Verification items for the finished model (mm, model axes). Round coordinates to 2 decimals unless told otherwise and drop trailing zeros. Order: outer loops, then holes, each group sorted by start corner. A loop starts at its lowest first (then second) coordinate and runs counter-clockwise, first axis right, second up. Notation, with made-up numbers: (10, 56.5) -> (18, 56.5) arc R30 cw to (18, 91.5) -> close; hole circle Ø11 at (58.25, 46.5). An arc over 180 degrees is marked (long way). Answer in a Markdown table with one row per item. Add a question column.
```python
from build123d import *

# Parameters (mm, degrees)
BOSS_EXTRUDE1_DEPTH = 3.175
CUT_EXTRUDE1_REACH  = 275.585
SKETCH2_W           = 1.6256
SKETCH2_H           = 4.7244


with BuildPart() as part:
    # Sketch1 → Boss-Extrude1 (new body)
    with BuildSketch(Plane(origin=(0, 0, 0), x_dir=(1, 0, 0), z_dir=(0, 1, 0))):
        Polygon((171.45, 101.6), (254, 101.6), (254, 0), (0, 0), (0, 101.6), (82.55, 101.6), (82.55, 76.2), (171.45, 76.2), align=None)
    extrude(amount=BOSS_EXTRUDE1_DEPTH)

    # Sketch2 → Cut-Extrude1 (cut, up to next)
    with BuildSketch(Plane(origin=(0, 3.175, 0), x_dir=(-1, 0, 0), z_dir=(0, 1, 0)), mode=Mode.PRIVATE) as cut_extrude1_sk1:
        with Locations((-97.742468943, -73.8378)):
            Rectangle(SKETCH2_W, SKETCH2_H)
    cut_extrude1_tool1 = extrude(cut_extrude1_sk1.sketch, amount=-CUT_EXTRUDE1_REACH, mode=Mode.PRIVATE) & part.part
    # Sketch2 → Cut-Extrude1 (cut, up to next)
    with BuildSketch(Plane(origin=(0, 3.175, 0), x_dir=(-1, 0, 0), z_dir=(0, 1, 0)), mode=Mode.PRIVATE) as cut_extrude1_sk2:
        Polygon((-113.996008389, -76.2), (-115.621608389, -76.2), (-115.621608389, -71.4756), (-113.996008389, -71.4756), (-113.996008389, -59.055), (-112.370408389, -59.055), (-112.370408389, -76.2), align=None)
    cut_extrude1_tool2 = extrude(cut_extrude1_sk2.sketch, amount=-CUT_EXTRUDE1_REACH, mode=Mode.PRIVATE) & part.part
    # Sketch2 → Cut-Extrude1 (cut, up to next)
    with BuildSketch(Plane(origin=(0, 3.175, 0), x_dir=(-1, 0, 0), z_dir=(0, 1, 0)), mode=Mode.PRIVATE) as cut_extrude1_sk3:
        with Locations((-139.191191611, -73.8378)):
            Rectangle(SKETCH2_W, SKETCH2_H)
    cut_extrude1_tool3 = extrude(cut_extrude1_sk3.sketch, amount=-CUT_EXTRUDE1_REACH, mode=Mode.PRIVATE) & part.part
    # Sketch2 → Cut-Extrude1 (cut, up to next)
    with BuildSketch(Plane(origin=(0, 3.175, 0), x_dir=(-1, 0, 0), z_dir=(0, 1, 0)), mode=Mode.PRIVATE) as cut_extrude1_sk4:
        with Locations((-156.257531057, -73.8378)):
            Rectangle(SKETCH2_W, SKETCH2_H)
    cut_extrude1_tool4 = extrude(cut_extrude1_sk4.sketch, amount=-CUT_EXTRUDE1_REACH, mode=Mode.PRIVATE) & part.part
    add(cut_extrude1_tool1.solids().sort_by_distance((97.742469, 3.175, -73.8378))[0], mode=Mode.SUBTRACT)
    add(cut_extrude1_tool2.solids().sort_by_distance((113.534383, 3.175, -68.969098))[0], mode=Mode.SUBTRACT)
    add(cut_extrude1_tool3.solids().sort_by_distance((139.191192, 3.175, -73.8378))[0], mode=Mode.SUBTRACT)
    add(cut_extrude1_tool4.solids().sort_by_distance((156.257531, 3.175, -73.8378))[0], mode=Mode.SUBTRACT)


solid = part.part
```
1) Cross-section at C-C, the plane x = 167.5. Record the boundary of the cut face in (y, z) (3 decimals), and give its area (3 significant figures).
2) Cross-section at A-A, the plane z = -95. Record the boundary of the cut face in (x, y) (3 decimals), and give its area (3 significant figures).
3) Depth check by flat-ended pin: P1, Ø0.5, axis at x = 156.5, y = 1.5, coming from the -Z side; P2, Ø1.5, axis at x = 118.5, y = 2.5, coming from the -Z side. Enter the tip coordinate at first touch or a pass-through.
4) Thickness scan on L1, parallel to X at y = 2.3, z = -78; L2, parallel to X at y = 3.05, z = -74.5; L3, parallel to Z at x = 107, y = 2.4. Record the ranges inside material, lowest first. Write a range as [from, to].
5) Cross-section at B-B, the plane y = 0.7. Record the boundary of the cut face in (x, z) (3 decimals), and give its area (3 significant figures).
Results below:
| question | item | result |
|---|---|---|
| 1 | outline | (0, -76.2) -> (3.175, -76.2) -> (3.175, 0) -> (0, 0) -> close |
| 1 | area | 242 mm² |
| 2 | outline | (0, 0) -> (82.55, 0) -> (82.55, 3.175) -> (0, 3.175) -> close; (171.45, 0) -> (254, 0) -> (254, 3.175) -> (171.45, 3.175) -> close |
| 2 | area | 524 mm² |
| 3 | P1 | z = -71.48 |
| 3 | P2 | z = -76.2 |
| 4 | L1 | [0, 82.55], [171.45, 254] |
| 4 | L2 | [0, 96.93], [98.56, 112.37], [115.62, 138.38], [140, 155.44], [157.07, 254] |
| 4 | L3 | [-76.2, 0] |
| 5 | outline | (0, -101.6) -> (82.55, -101.6) -> (82.55, -76.2) -> (96.93, -76.2) -> (96.93, -71.476) -> (98.555, -71.476) -> (98.555, -76.2) -> (112.37, -76.2) -> (112.37, -59.055) -> (113.996, -59.055) -> (113.996, -71.476) -> (115.622, -71.476) -> (115.622, -76.2) -> (138.378, -76.2) -> (138.378, -71.476) -> (140.004, -71.476) -> (140.004, -76.2) -> (155.445, -76.2) -> (155.445, -71.476) -> (157.07, -71.476) -> (157.07, -76.2) -> (171.45, -76.2) -> (171.45, -101.6) -> (254, -101.6) -> (254, 0) -> (0, 0) -> close |
| 5 | area | 23,500 mm² |
